Geometry: see drawing. Coordinates: mm, zero at the bounding-box minimum. A direction names the side the tool comes from. Coordinates: 2 decimals unless noted, no trailing zeros. Write each loop counter-clockwise with the first axis right and the second up, starting at its lowest first coordinate (ties: lowest second). Pieces come first, ordered by that corner, then holes.
1) Set-up query: the marked faces 4 and 5. Return all of +Z, -Z, +X, -X, +Y, -Y with unobstructed straight access to the full face (end or side cutting, diameter ignored); none if empty.
2) Draft query along Z for the marked faces 1, 2 and 3. Return one class per face: pulls with the +Z half, pulls with the -Z half, needs draft (parallel to the pull), parting line crosses it, or undercut.
3) Pin query (flat end, axial travel): pin 1 Ø18.5 at (x, z) = (22, 60) entering from -Y; pin 2 Ø10 at (x, z) = (71, 65) entering from -Y. Return the tip coordinate at first contact, or that it passes through.
4) Section query B-B (x = 100). Output: boundary loops of the cut face in (y, z).
5) Line query: L1, parallel to Z at x = 31.5, y = 62; L2, parallel to Y at x = 149.5, z = 35; L3, parallel to Y at x = 145.5, z = 95. Output: solid intervals per line, ascending.
6) Section query D-D (x = 182). Output: boundary loops of the cut face in (y, z), then the cut area to 3 significant figures.
7) Section query A-A (y = 47). Output: boundary loops of the cut face in (x, z).
8) Section query C-C (y = 68). Output: boundary loops of the cut face in (x, z).
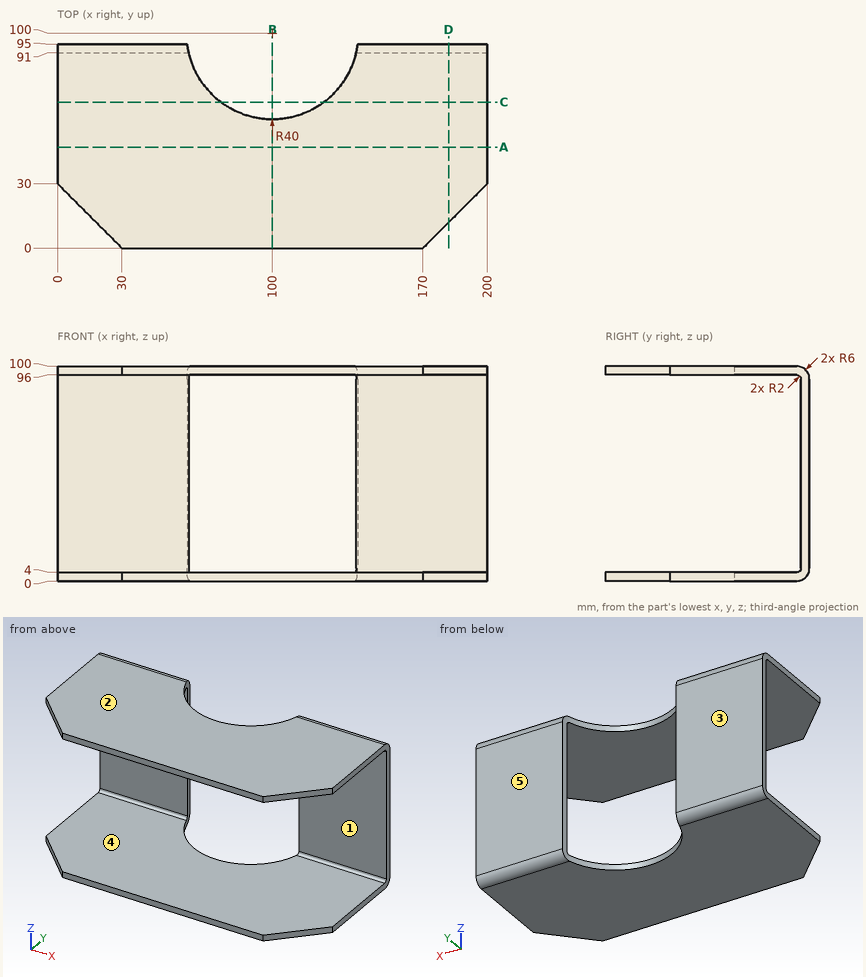
Answer:
1. face 4: +X, -X, -Y
1. face 5: +Z, -Z, +X, -X, +Y
2. face 1: undercut
2. face 2: pulls with the +Z half
2. face 3: needs draft
3. pin 1: stops at y = 91
3. pin 2: passes through
4. outline: (0, 0) - (60, 0) - (60, 4) - (0, 4) - close; (0, 96) - (60, 96) - (60, 100) - (0, 100) - close
5. L1: z = 0 to 4, 96 to 100
5. L2: y = 91 to 95
5. L3: y = 90.73 to 94.92
6. outline: (12, 0) - (89, 0) arc R6 ccw to (95, 6) - (95, 94) arc R6 ccw to (89, 100) - (12, 100) - (12, 96) - (89, 96) arc R2 cw to (91, 94) - (91, 6) arc R2 cw to (89, 4) - (12, 4) - close
6. area: 1,020 mm2
7. outline: (0, 0) - (200, 0) - (200, 4) - (0, 4) - close; (0, 96) - (200, 96) - (200, 100) - (0, 100) - close
8. outline: (0, 0) - (76, 0) - (76, 4) - (0, 4) - close; (0, 96) - (76, 96) - (76, 100) - (0, 100) - close; (124, 0) - (200, 0) - (200, 4) - (124, 4) - close; (124, 96) - (200, 96) - (200, 100) - (124, 100) - close
